CAD build for the part. Positions are in the model's coordinates, mm. A direction names the side the tool comes from. Coordinates: 2 decimals unless noted, no trailing zeros. Loops run counter-clockwise (first coordinate to the right, second up) from the corner with the lowest first, then second, coordinate; pieces in that order, holes last. Notation, with made-up numbers: (29, 70) -> (82, 70) arc R12 ccw to (82, 85) -> close; hole circle Ø4 at (-30.75, 65). An arc over 180 degrees is marked (long way). Answer as a JSON object with one key per item and string values. Group by question number.
from build123d import *

# Parameters (mm, degrees)
BOSS_EXTRUDE1_DEPTH     = 35
CUT_EXTRUDE1_DEPTH      = 1
CUT_EXTRUDE1_DEPTH_BACK = 181
CUT_EXTRUDE2_DEPTH      = 70
SKETCH9_W               = 70
SKETCH9_H               = 16
CUT_EXTRUDE4_DEPTH      = 70
BOSS_EXTRUDE2_DEPTH     = 28


with BuildPart() as part:
    # Sketch2 → Boss-Extrude1 (new body, symmetric)
    with BuildSketch(Plane.XY):
        Polygon((-72, 38), (-72, -7), (64, -7), (64, 38), (90, 38), (90, -38), (-90, -38), (-90, 38), align=None)
    extrude(amount=BOSS_EXTRUDE1_DEPTH, both=True)

    # Sketch3 → Cut-Extrude1 (cut, two sides)
    with BuildSketch(Plane(origin=(90, 0, 0), x_dir=(0, 0, -1), z_dir=(1, 0, 0))) as cut_extrude1_sk:
        Polygon((16, -38), (16, -19), (13, -19), (13, 3), (-13, 3), (-13, -19), (-16, -19), (-16, -38), align=None)
    extrude(amount=CUT_EXTRUDE1_DEPTH, mode=Mode.SUBTRACT)
    extrude(cut_extrude1_sk.sketch, amount=-CUT_EXTRUDE1_DEPTH_BACK, mode=Mode.SUBTRACT)

    # Sketch5 → Cut-Extrude2 (cut)
    with BuildSketch(Plane.XY.offset(35)):
        with BuildLine():
            Line((-90, 24), (-86, 24))
            ThreePointArc((-86, 24), (-81.899494937, 33.899494937), (-72, 38))
            Line((-72, 38), (-90, 38))
            Line((-90, 38), (-90, 24))
        make_face()
    extrude(amount=-CUT_EXTRUDE2_DEPTH, mode=Mode.SUBTRACT)

    # Sketch9 → Cut-Extrude4 (cut)
    with BuildSketch(Plane(origin=(90, 0, 0), x_dir=(0, 0, -1), z_dir=(1, 0, 0))):
        with Locations((0, 30)):
            Rectangle(SKETCH9_W, SKETCH9_H)
    extrude(amount=-CUT_EXTRUDE4_DEPTH, mode=Mode.SUBTRACT)

    # Sketch10 → Boss-Extrude2 (add)
    with BuildSketch(Plane(origin=(90, 0, 0), x_dir=(0, 0, -1), z_dir=(1, 0, 0))):
        with BuildLine():
            Line((-16, 22), (16, 22))
            ThreePointArc((16, 22), (0, 38), (-16, 22))
        make_face()
    extrude(amount=-BOSS_EXTRUDE2_DEPTH)


solid = part.part
Item 1: Band-saw the part on B-B, the plane x = 41. List the corners of the cut face in (y, z).
Item 2: Band-saw the part on A-A, the plane y = -9.5. List the corners of the cut face in (x, z).
Item 3: 3-axis set-ups, long thin cutter, end or side, ignore diameter. For faces 4 (the flat face through (-72, 16, 0)), 5 (the flat face through (64, 7, 0)), 6 (the flat face through (-81, 3, 0)): which of +Z, -Z, +X, -X, +Y, -Y reach the whole face in a straight line?
Item 4: Band-saw the part on C-C, the plane z = 0. List the corners of the cut face in (x, y).
Item 5: Pull direction Z, two halves, no side cores. Call faces 1 (the flat face through (77, 22, -25)), 2 (the flat face through (1, -29, -16)), 3 (the cylindrical face through (76, 38, 0)): +Z half, -Z half, draft (parallel to the pull), parting line (faces both ways), or undercut.
Item 6: Drill centre lines: L1, parallel to X at y = 11, z = 5.5; L2, parallel to Z at x = 44.5, y = -20; L3, parallel to Z at x = 70, y = -16.5. Where is each one in solid material? Low to high.
Item 7: Band-saw the part on D-D, the plane z = -23.5. List the corners of the cut face in (x, y), and give its area (3 significant figures).
Item 8: Flat gauge pins, fed straight in: P1, Ø8, axis at y = 30, z = -4.5, coming from the -X side; P2, Ø6.5, axis at x = 21.5, z = 27, coming from the +Y side; P3, Ø1.2, axis at x = -88.5, z = 0.5, coming from the +Y side. Where does each tip first touch, or does it go through?
Reply:
{
 "1": {"outline": "(-38, -35) -> (-7, -35) -> (-7, -13) -> (-19, -13) -> (-19, -16) -> (-38, -16) -> close; (-38, 16) -> (-19, 16) -> (-19, 13) -> (-7, 13) -> (-7, 35) -> (-38, 35) -> close"},
 "2": {"outline": "(-90, -35) -> (90, -35) -> (90, -13) -> (-90, -13) -> close; (-90, 13) -> (90, 13) -> (90, 35) -> (-90, 35) -> close"},
 "3": {"face 4": "+Z, -Z, +Y", "face 5": "+Z, -Z", "face 6": "+X, -X, -Y"},
 "4": {"outline": "(-90, 3) -> (-72, 3) -> (-72, 38) arc R14 ccw to (-86, 24) -> (-90, 24) -> close; (62, 22) -> (64, 22) -> (64, 3) -> (90, 3) -> (90, 38) -> (62, 38) -> close"},
 "5": {"face 1": "draft", "face 2": "undercut", "face 3": "parting line"},
 "6": {"L1": "-90 to -72, 64 to 90", "L2": "-35 to -16, 16 to 35", "L3": "-35 to -13, 13 to 35"},
 "7": {"outline": "(-90, -38) -> (90, -38) -> (90, 22) -> (64, 22) -> (64, -7) -> (-72, -7) -> (-72, 38) arc R14 ccw to (-86, 24) -> (-90, 24) -> close", "area": "7,050 mm²"},
 "8": {"P1": "x = -85.86", "P2": "y = -7", "P3": "y = 24"}
}
